```python
from build123d import *

# Parameters (mm, degrees)
BASE_FLANGE1_DEPTH = 10
SKETCH4_R          = 1.5
CUT_EXTRUDE1_DEPTH = 27.149638759


# Sheet-metal steps are written as plain solids
with BuildPart() as part:
    # Sketch1 → Base-Flange1 (new body)
    with BuildSketch(Plane(origin=(0, 0, 0), x_dir=(1, 0, 0), z_dir=(0, 1, 0))):
        with BuildLine():
            Line((0, 0), (6.757359313, 0))
            ThreePointArc((6.757359313, 0), (7.90540961, -0.228361402), (8.878679656, -0.878679656))
            Line((8.878679656, -0.878679656), (20.727922061, -12.727922061))
            Line((20.727922061, -12.727922061), (20.02081528, -13.435028843))
            Line((20.02081528, -13.435028843), (8.171572875, -1.585786438))
            ThreePointArc((8.171572875, -1.585786438), (7.522726178, -1.152240935), (6.757359313, -1))
            Line((6.757359313, -1), (0, -1))
            Line((0, -1), (0, 0))
        make_face()
    extrude(amount=BASE_FLANGE1_DEPTH)

    # Sketch4 → Cut-Extrude1 (cut, through all)
    with BuildSketch(Plane(origin=(3.292893219, 0, -3.292893219), x_dir=(0.7071067811865465, 0, 0.7071067811865486), z_dir=(-0.7071067811865486, 0, 0.7071067811865465))):
        with Locations((19.656854249, 5)):
            Circle(SKETCH4_R)
    extrude(amount=-CUT_EXTRUDE1_DEPTH, mode=Mode.SUBTRACT)


solid = part.part
```
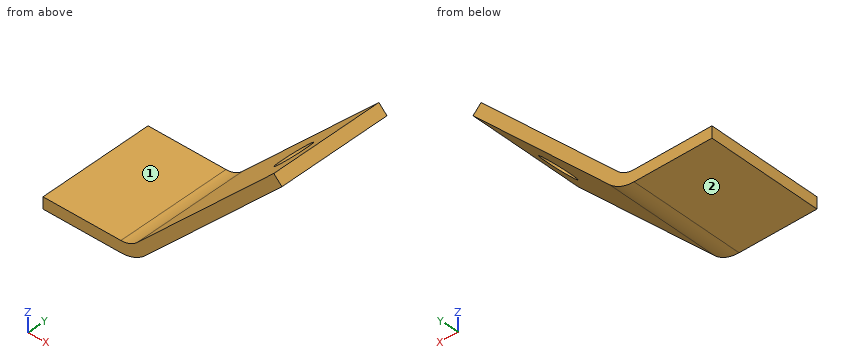
The listing builds one solid part. Answer for the finished solid, in the listing's coordinates (mm). Face numbers are marked on the shaded views. A direction names the side the tool comes from. Give positions to 0.01 mm unless a question says otherwise; leave off trailing zeros. Order: outer loops, then holes, each group sorted by start corner. A loop starts at its lowest first (then second) coordinate and runs counter-clockwise, first axis right, second up. Notation, with made-up numbers: (-11, -20) - (17, -20) arc R19 cw to (17, -4) - close; hole circle Ø9 at (6.25, 63.5). An arc over 180 degrees is marked (long way). Use one line per item in the form item = value. Start each with the question number.
(1) A cutting plane is placed at D-D, the plane z = 12. Write down the section's boundary in (x, y), then the cut area to 3 significant figures.
(2) A cutting plane is placed at C-C, the plane x = 6. Write down the section's boundary in (y, z), then the cut area to 3 significant figures.
(3) Flat-ended cylindrical pins translate along their axes: pin 1 Ø5.5 at (x, y) = (4.5, 4) entering from +Z; pin 2 Ø3 at (y, z) = (1.5, 8) entering from +X; pin 3 Ø5 at (y, z) = (6.5, 7.5) entering from +X. Find the tip coordinate at first contact, or state that the pin passes through.
(4) For the marked faces 1 and 2, determine the directions among +Z, -Z, +X, -X, +Y, -Y from which every point of the face is accessible in a straight line to the end or side of a thin tool.
(5) A cutting plane is placed at B-B, the plane y = 1.75. Write down the section's boundary in (x, z), then the cut area to 3 significant figures.
(6) A cutting plane is placed at A-A, the plane y = 4. Write down the section's boundary in (x, z).
(7) Consider line 1 (Z direction, x = 4, y = 1.5); line 2 (X direction, y = 4.5, z = 5); line 3 (Z direction, x = 18.25, y = 8). Determine where each line is inside the solid, lowest interval first. Write a range as from..to.
Ans:
q1.outline = (18.59, 0) - (20, 0) - (20, 10) - (18.59, 10) - close
q1.area = 14.1 mm^2
q2.outline = (0, 0) - (10, 0) - (10, 1) - (0, 1) - close
q2.area = 10.0 mm^2
q3.pin_1 = 1.06
q3.pin_2 = 17.5
q3.pin_3 = 18
q4.face_1 = +Z, -X, +Y, -Y
q4.face_2 = -Z, +X, -X, +Y, -Y
q5.outline = (0, 0) - (6.76, 0) arc R3 ccw to (8.88, 0.88) - (20.73, 12.73) - (20.02, 13.44) - (8.17, 1.59) arc R2 cw to (6.76, 1) - (0, 1) - close
q5.area = 25.5 mm^2
q6.outline = (0, 0) - (6.76, 0) arc R3 ccw to (8.88, 0.88) - (17.11, 9.11) - (16.4, 9.82) - (8.17, 1.59) arc R2 cw to (6.76, 1) - (0, 1) - close; (17.98, 11.4) - (18.69, 10.69) - (20.73, 12.73) - (20.02, 13.44) - close
q7.line_1 = 0..1
q7.line_2 = 11.59..13
q7.line_3 = 10.25..11.66
